Could you check a few things on this model? Use its own coordinates, in mm. A direction names the side the tool comes from. Round coordinates to 2 decimals unless told otherwise and drop trailing zeros. Order: outer loops, then holes, each group sorted by start corner. A loop starts at its lowest first (then second) coordinate and runs counter-clockwise, first axis right, second up. Notation, with made-up numbers: (1, 81) - (31, 81) arc R12 cw to (31, 94) - close; hole circle Ø5 at (78, -30.75). An arc over 180 degrees is marked (long way). Return JSON: item names as keys, results as strings. Group by question number.
from build123d import *

# Parameters (mm, degrees)
SKETCH1_R               = 104.60742403
BOSS_EXTRUDE6_DEPTH     = 50.8
SKETCH4_R               = 54.991
CUT_EXTRUDE2_DEPTH      = 109.982
CUT_EXTRUDE2_DRAFT      = -20
SKETCH6_R               = 11.049
CUT_EXTRUDE4_DEPTH      = 22.86
CUT_EXTRUDE5_DEPTH      = 8.89
CUT_EXTRUDE5_DEPTH_BACK = 13.97
SKETCH8_R               = 102.235
SKETCH8_R_2             = 56.007
CUT_EXTRUDE6_DEPTH      = 8.89
CUT_EXTRUDE6_DEPTH_BACK = 11.684
SKETCH9_R               = 102.235
SKETCH9_R_2             = 56.007
CUT_EXTRUDE7_DEPTH      = 2.54
CUT_EXTRUDE7_DEPTH_BACK = 2.54
SKETCH10_R              = 6.35


with BuildPart() as part:
    # Sketch1 → Boss-Extrude6 (new body)
    with BuildSketch(Plane.XY):
        with Locations((-38.924588073, 36.746668339)):
            Circle(SKETCH1_R)
    extrude(amount=BOSS_EXTRUDE6_DEPTH)


with BuildPart() as cut_extrude2_tool:
    # Sketch4 → Cut-Extrude2 (with draft: the straight prism first)
    with BuildSketch(Plane.XY.offset(50.8)):
        with Locations((-38.924588073, 36.746668339)):
            Circle(SKETCH4_R)
    extrude(amount=-CUT_EXTRUDE2_DEPTH)
    # Cut-Extrude2: the draft: its side faces are tilted about the plane it starts from
    cut_extrude2_sides = [cut_extrude2_tool.faces().sort_by_distance(p)[0] for p in [
        (-93.915588073, 36.746668339, -4.191),
    ]]
    draft(cut_extrude2_sides, Plane.XY.offset(50.8), CUT_EXTRUDE2_DRAFT)


with BuildPart() as part_1:
    add(part.part)

    # Cut-Extrude2: cut by cut_extrude2_tool
    add(cut_extrude2_tool.part, mode=Mode.SUBTRACT)

    # Sketch6 → Cut-Extrude4 (cut)
    with BuildSketch(Plane.XY.offset(50.8)):
        with Locations((23.28775176, 101.513937691)):
            Circle(SKETCH6_R)
        with Locations((-26.662993645, 125.711985788)):
            Circle(SKETCH6_R)
        with Locations((-38.924588073, 104.485307018)):
            Circle(SKETCH6_R)
        with Locations((-51.165531001, 125.711985788)):
            Circle(SKETCH6_R)
        with Locations((0.891184754, 91.548378206)):
            Circle(SKETCH6_R)
        with Locations((3.464782634, 115.916167792)):
            Circle(SKETCH6_R)
        with Locations((49.475497868, 52.57699406)):
            Circle(SKETCH6_R)
        with Locations((25.498685648, 57.679058867)):
            Circle(SKETCH6_R)
        with Locations((41.90379742, 75.880291878)):
            Circle(SKETCH6_R)
        with Locations((41.897415755, -2.406595944)):
            Circle(SKETCH6_R)
        with Locations((25.498685648, 15.814277811)):
            Circle(SKETCH6_R)
        with Locations((49.469116204, 20.896701874)):
            Circle(SKETCH6_R)
        with Locations((3.448075219, -42.434969762)):
            Circle(SKETCH6_R)
        with Locations((0.891184754, -18.055041529)):
            Circle(SKETCH6_R)
        with Locations((23.271044345, -28.03273966)):
            Circle(SKETCH6_R)
        with Locations((-51.186182501, -52.218649111)):
            Circle(SKETCH6_R)
        with Locations((-38.924588073, -30.991970341)):
            Circle(SKETCH6_R)
        with Locations((-26.683645145, -52.218649111)):
            Circle(SKETCH6_R)
        with Locations((-101.136927905, -28.020601013)):
            Circle(SKETCH6_R)
        with Locations((-78.740360899, -18.055041529)):
            Circle(SKETCH6_R)
        with Locations((-81.313958779, -42.422831115)):
            Circle(SKETCH6_R)
        with Locations((-127.324674013, 20.916342618)):
            Circle(SKETCH6_R)
        with Locations((-103.347861794, 15.814277811)):
            Circle(SKETCH6_R)
        with Locations((-119.752973565, -2.3869552)):
            Circle(SKETCH6_R)
        with Locations((-119.746591901, 75.899932621)):
            Circle(SKETCH6_R)
        with Locations((-103.347861794, 57.679058867)):
            Circle(SKETCH6_R)
        with Locations((-127.318292349, 52.596634803)):
            Circle(SKETCH6_R)
        with Locations((-81.297251365, 115.928306439)):
            Circle(SKETCH6_R)
        with Locations((-78.740360899, 91.548378206)):
            Circle(SKETCH6_R)
        with Locations((-101.120220491, 101.526076338)):
            Circle(SKETCH6_R)
    extrude(amount=-CUT_EXTRUDE4_DEPTH, mode=Mode.SUBTRACT)

    # Sketch8 → Cut-Extrude5 (cut, two sides: drawn at the far end of the back side and taken through both)
    with BuildSketch(Plane.XY.offset(13.97).offset(-CUT_EXTRUDE5_DEPTH_BACK)):
        with Locations((-38.924588073, 36.746668339)):
            Circle(SKETCH8_R)
        with Locations((-38.924588073, 36.746668339)):
            Circle(SKETCH8_R_2, mode=Mode.SUBTRACT)
    extrude(amount=CUT_EXTRUDE5_DEPTH + CUT_EXTRUDE5_DEPTH_BACK, mode=Mode.SUBTRACT)

    # Sketch9 → Cut-Extrude6 (cut, two sides: drawn at the far end of the back side and taken through both)
    with BuildSketch(Plane(origin=(0, 0, 36.83), x_dir=(-1, 0, 0), z_dir=(0, 0, -1)).offset(-CUT_EXTRUDE6_DEPTH_BACK)):
        with Locations(Location((38.924588073, 36.746668339, 0), (0, 0, 180))):
            Circle(SKETCH9_R)
        with Locations(Location((38.924588073, 36.746668339, 0), (0, 0, 180))):
            Circle(SKETCH9_R_2, mode=Mode.SUBTRACT)
    extrude(amount=CUT_EXTRUDE6_DEPTH + CUT_EXTRUDE6_DEPTH_BACK, mode=Mode.SUBTRACT)

    # Sketch10 → Cut-Extrude7 (cut, two sides: drawn at the far end of the back side and taken through both)
    with BuildSketch(Plane.XY.offset(25.4).offset(-CUT_EXTRUDE7_DEPTH_BACK)):
        with Locations((37.275304422, 36.618668929)):
            Circle(SKETCH10_R)
        with Locations((-15.499260995, -35.763289952)):
            Circle(SKETCH10_R)
        with Locations((-100.646832236, -7.938950998)):
            Circle(SKETCH10_R)
        with Locations((-15.25579165, 109.177518644)):
            Circle(SKETCH10_R)
        with Locations((-100.496359905, 81.639395071)):
            Circle(SKETCH10_R)
    extrude(amount=CUT_EXTRUDE7_DEPTH + CUT_EXTRUDE7_DEPTH_BACK, mode=Mode.SUBTRACT)


solid = part_1.part
1) For faces 5 (the cylindrical face through (-16.63, 102.98, 25.36)), 6 (the cylindrical face through (9.345, -56.058, 25.044)), 7 (the flat face through (-92, 14, 48.514)), 8 (the cylindrical face through (-47.068, -23.525, 49.673)), which set-ups out of +Z, -Z, +X, -X, +Y, -Y let a thin tool reach every point of the face, with its end or its side?
2) If I drill on line 1 along Y through (x, z) = (-40.5, 3); line 2 along Y through (x, z) = (-78.5, 31.5); line 3 along X through (y, z) = (66, 31.5), over which ranges is the centre line in solid material (lowest first)? Write a range as from..to.
3) Will these pins go through, and if not, where does the flat tip stop? pin 1 (4 mm diameter, centred on y = 39.5, z = 44, fed in from -X); pin 2 (10 mm diameter, centred on y = 114, z = 24, fed in from -X); pin 3 (5 mm diameter, centred on y = 4.5, z = 18.5, fed in from +X).
4) I want a section at B-B, the plane y = -48.5. List the corners of the cut face in (x, z) for me.
5) I want a section at A-A, the plane x = 49. List the corners of the cut face in (y, z) for me, plus the area to 3 significant figures.
6) I want a section at C-C, the plane z = 45. List the corners of the cut face in (x, y) for me (3 decimals), plus the area to 3 significant figures.
7) I want a section at D-D, the plane x = -103. Give the number of separate pieces and of enclosed holes in the cut face, plus the area to 3 significant figures.
8) We'd pull the mould along Z, two halves only. Please class faces 1 (the flat face through (5, 81, 27.94)), 2 (the flat face through (-2, 38, 0)), 3 (the cylindrical face through (31.439, 66.996, 49.673)), 4 (the conical face through (-2.24, 21.54, 8.82)): +Z half, -Z half, draft (parallel to the pull), parting line (faces both ways), or undercut.
Outcome:
{
 "1": {"face 5": "-Z", "face 6": "+Z, -Z", "face 7": "none", "face 8": "+Z"},
 "2": {"line 1": "-67.85..-65.48, -19.24..-0.81, 74.31..92.73, 138.97..141.34", "line 2": "-60.09..-57.52, -2.88..9.64, 63.85..76.38, 131.01..133.58", "line 3": "-139.36..-136.88, -86.68..-76.94, -0.91..8.84, 59.04..61.51"},
 "3": {"pin 1": "x = -143.53", "pin 2": "x = -114.57", "pin 3": "x = 61.36"},
 "4": {"outline": "(-99.55, 0) - (-95.36, 0) - (-95.36, 22.86) - (17.51, 22.86) - (17.51, 0) - (21.7, 0) - (21.7, 50.8) - (12.68, 50.8) - (12.68, 48.51) - (17.51, 48.51) - (17.51, 27.94) - (-95.36, 27.94) - (-95.36, 48.51) - (-90.54, 48.51) - (-90.54, 50.8) - (-99.55, 50.8) - close; (-72.09, 48.51) - (-61.59, 48.51) - (-61.59, 50.8) - (-72.09, 50.8) - close; (-40.78, 48.51) - (-37.09, 48.51) - (-37.09, 50.8) - (-40.78, 50.8) - close; (-16.28, 48.51) - (-5.79, 48.51) - (-5.79, 50.8) - (-16.28, 50.8) - close"},
 "5": {"outline": "(-19.93, 0) - (-15.42, 0) - (-15.42, 22.86) - (88.91, 22.86) - (88.91, 0) - (93.42, 0) - (93.42, 50.8) - (84.35, 50.8) - (84.35, 48.51) - (88.91, 48.51) - (88.91, 27.94) - (-15.42, 27.94) - (-15.42, 48.51) - (-10.87, 48.51) - (-10.87, 50.8) - (-19.93, 50.8) - close; (6.06, 48.51) - (9.86, 48.51) - (9.86, 50.8) - (6.06, 50.8) - close; (31.94, 48.51) - (41.54, 48.51) - (41.54, 50.8) - (31.94, 50.8) - close; (63.62, 48.51) - (67.41, 48.51) - (67.41, 50.8) - (63.62, 50.8) - close", "area": "1,050 mm^2"},
 "6": {"outline": "circle Ø209.215 at (-38.925, 36.747); circle Ø112.014 at (-38.925, 36.747); hole circle Ø204.47 at (-38.925, 36.747); hole circle Ø105.76 at (-38.925, 36.747)", "area": "2,610 mm^2"},
 "7": {"separate pieces": "6", "enclosed holes": "0", "area": "1,160 mm^2"},
 "8": {"face 1": "undercut", "face 2": "-Z half", "face 3": "draft", "face 4": "+Z half"}
}
